from build123d import *

# Parameters (mm, degrees)
SKETCH1_W           = 155
SKETCH1_H           = 20
BOSS_EXTRUDE1_DEPTH = 40
CUT_EXTRUDE1_DEPTH  = 3
SKETCH4_W           = 78
SKETCH4_H           = 38
BOSS_EXTRUDE2_DEPTH = 20
FILLET1_R           = 5
SHELL2_START        = -10
SHELL2_DEPTH        = 18
SHELL2_START_2      = 2
SHELL2_2_DEPTH      = 3
CUT_EXTRUDE3_DEPTH  = 112.759787043
CUT_EXTRUDE4_REACH  = 110.311
SKETCH8_R           = 8
SKETCH9_R           = 2.05
CUT_EXTRUDE5_DEPTH  = 1.1


with BuildPart() as part:
    # Sketch1 → Boss-Extrude1 (new body)
    with BuildSketch(Plane(origin=(0, 0, 0), x_dir=(1, 0, 0), z_dir=(0, 1, 0))):
        Rectangle(SKETCH1_W, SKETCH1_H)
    extrude(amount=BOSS_EXTRUDE1_DEPTH)

    # Sketch2 → Cut-Extrude1 (cut)
    with BuildSketch(Plane.XZ):
        with BuildLine():
            Line((-71, -8), (71, -8))
            ThreePointArc((71, -8), (74.535533906, -6.535533906), (76, -3))
            Line((76, -3), (76, 3))
            ThreePointArc((76, 3), (74.535533906, 6.535533906), (71, 8))
            Line((71, 8), (-71, 8))
            ThreePointArc((-71, 8), (-74.535533906, 6.535533906), (-76, 3))
            Line((-76, 3), (-76, -3))
            ThreePointArc((-76, -3), (-74.535533906, -6.535533906), (-71, -8))
        make_face()
    extrude(amount=-CUT_EXTRUDE1_DEPTH, mode=Mode.SUBTRACT)

    # Sketch4 → Boss-Extrude2 (add)
    with BuildSketch(Plane.XY.offset(10)):
        with Locations((0, 59)):
            Rectangle(SKETCH4_W, SKETCH4_H)
    extrude(amount=-BOSS_EXTRUDE2_DEPTH)

    # Fillet1
    fillet1_edges = [part.edges().sort_by_distance(p)[0] for p in [
        (-77.5, 40, 0),
        (77.5, 40, 0),
        (-39, 78, 0),
        (39, 78, 0),
    ]]
    fillet(fillet1_edges, radius=FILLET1_R)

    # Shell2: read off the stored shape, not the designer's step
    # Shell2 outline → Shell2 (cut)
    with BuildSketch(Plane.XY.offset(SHELL2_START)):
        with BuildLine():
            Line((-75.5, 35), (-75.5, 5))
            Line((-75.5, 5), (75.5, 5))
            Line((75.5, 5), (75.5, 35))
            ThreePointArc((75.5, 35), (74.621320344, 37.121320344), (72.5, 38))
            Line((72.5, 38), (37, 38))
            Line((37, 38), (37, 73))
            ThreePointArc((37, 73), (36.121320344, 75.121320344), (34, 76))
            Line((34, 76), (-34, 76))
            ThreePointArc((-34, 76), (-36.121320344, 75.121320344), (-37, 73))
            Line((-37, 73), (-37, 38))
            Line((-37, 38), (-72.5, 38))
            ThreePointArc((-72.5, 38), (-74.621320344, 37.121320344), (-75.5, 35))
        make_face()
    extrude(amount=SHELL2_DEPTH, mode=Mode.SUBTRACT)

    # Shell2 2 outline → Shell2 2 (cut)
    with BuildSketch(Plane(origin=(0, 0, 0), x_dir=(1, 0, 0), z_dir=(0, 1, 0)).offset(SHELL2_START_2)):
        with BuildLine():
            Line((75.5, 10), (71, 10))
            ThreePointArc((71, 10), (73.394439545, 9.577739678), (75.5, 8.361902647))
            Line((75.5, 8.361902647), (75.5, 10))
        make_face()
        with BuildLine():
            ThreePointArc((-75.5, 8.361902647), (-73.394439545, 9.577739678), (-71, 10))
            Line((-71, 10), (-75.5, 10))
            Line((-75.5, 10), (-75.5, 8.361902647))
        make_face()
    extrude(amount=SHELL2_2_DEPTH, mode=Mode.SUBTRACT)

    # Sketch7 → Cut-Extrude3 (cut, through all)
    with BuildSketch(Plane.XY.offset(10)):
        with BuildLine():
            Line((-32.75, 18.5), (-32.75, 25.5))
            ThreePointArc((-32.75, 25.5), (-32.5, 25.75), (-32.25, 25.5))
            Line((-32.25, 25.5), (-32.25, 18.5))
            ThreePointArc((-32.25, 18.5), (-32.5, 18.25), (-32.75, 18.5))
        make_face()
        with BuildLine():
            Line((-31.75, 19.5), (-31.75, 24.5))
            ThreePointArc((-31.75, 24.5), (-31.5, 24.75), (-31.25, 24.5))
            Line((-31.25, 24.5), (-31.25, 19.5))
            ThreePointArc((-31.25, 19.5), (-31.5, 19.25), (-31.75, 19.5))
        make_face()
        with BuildLine():
            Line((-30.75, 20.5), (-30.75, 23.5))
            ThreePointArc((-30.75, 23.5), (-30.5, 23.75), (-30.25, 23.5))
            Line((-30.25, 23.5), (-30.25, 20.5))
            ThreePointArc((-30.25, 20.5), (-30.5, 20.25), (-30.75, 20.5))
        make_face()
        with BuildLine():
            Line((-33.25, 19.5), (-33.25, 24.5))
            ThreePointArc((-33.25, 24.5), (-33.5, 24.75), (-33.75, 24.5))
            Line((-33.75, 24.5), (-33.75, 19.5))
            ThreePointArc((-33.75, 19.5), (-33.5, 19.25), (-33.25, 19.5))
        make_face()
        with BuildLine():
            Line((-34.25, 20.5), (-34.25, 23.5))
            ThreePointArc((-34.25, 23.5), (-34.5, 23.75), (-34.75, 23.5))
            Line((-34.75, 23.5), (-34.75, 20.5))
            ThreePointArc((-34.75, 20.5), (-34.5, 20.25), (-34.25, 20.5))
        make_face()
    cut_extrude3 = extrude(amount=-CUT_EXTRUDE3_DEPTH, mode=Mode.SUBTRACT)

    # Mirror1: Cut-Extrude3 across plane
    add(cut_extrude3.mirror(Plane(origin=(0, 0, 0), x_dir=(0, 0, 1), z_dir=(1, 0, 0))), mode=Mode.SUBTRACT)

    # Sketch8 → Cut-Extrude4 (cut, up to next)
    with BuildSketch(Plane.XZ.offset(-3), mode=Mode.PRIVATE) as cut_extrude4_sk1:
        with Locations(Location((0, 0, 0), (0, 0, 90))):
            Circle(SKETCH8_R)
    cut_extrude4_tool1 = extrude(cut_extrude4_sk1.sketch, amount=-CUT_EXTRUDE4_REACH, mode=Mode.PRIVATE) & part.part
    add(cut_extrude4_tool1.solids().sort_by_distance((0, 3, 0))[0], mode=Mode.SUBTRACT)

    # Sketch9 → Cut-Extrude5 (cut)
    with BuildSketch(Plane.XZ.offset(-3)):
        with Locations(Location((70.75, 2.75, 0), (0, 0, 270))):
            Circle(SKETCH9_R)
        with Locations(Location((66.25, 2.75, 0), (0, 0, 270))):
            Circle(SKETCH9_R)
        with Locations(Location((66.25, -2.75, 0), (0, 0, 270))):
            Circle(SKETCH9_R)
        with Locations(Location((70.75, -2.75, 0), (0, 0, 270))):
            Circle(SKETCH9_R)
    cut_extrude5 = extrude(amount=-CUT_EXTRUDE5_DEPTH, mode=Mode.SUBTRACT)

    # Mirror2: Cut-Extrude5 across plane
    add(cut_extrude5.mirror(Plane(origin=(0, 0, 0), x_dir=(0, 0, 1), z_dir=(1, 0, 0))), mode=Mode.SUBTRACT)


solid = part.part
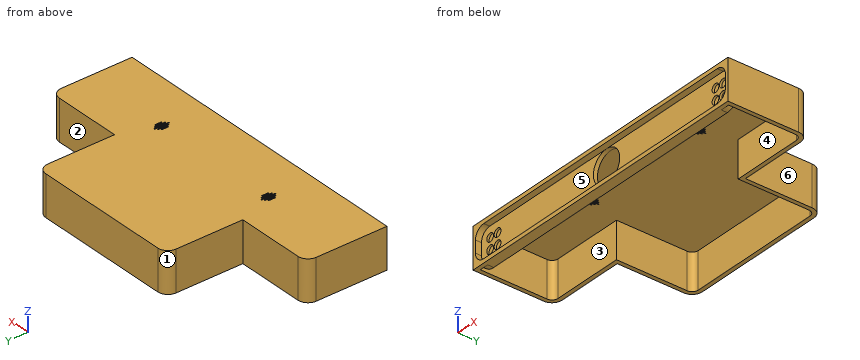
Geometry check sheet. Reference: the model listing, model coordinates, mm. Face numbers are marked on the shaded views. A direction names the side the tool comes from. Round coordinates to 2 decimals unless told otherwise and drop trailing zeros. Loops run counter-clockwise (first coordinate to the right, second up) from the corner with the lowest first, then second, coordinate; pieces in that order, holes last. Notation, with made-up numbers: (-24.5, 45.25) - (1.5, 45.25) arc R21 ccw to (1.5, 50.25) - close; hole circle Ø10 at (46, 10.25). An arc over 180 degrees is marked (long way). One line per question, with ' | ' between items. Start each with the question number.
1. Scan lines: line 1 (X direction, y = 18, z = -8); line 2 (Y direction, x = 52, z = -3.5); line 3 (X direction, y = 69, z = -6). Record each from-to range of solid material in increasing order. Write a range as [from, to].
2. Tool access check on the marked faces 4, 5 and 6. Record the directions out of +Z, -Z, +X, -X, +Y, -Y that give a thin tool (end or side, any length) a straight path to the whole face; none if there is none.
3. Draft check along X on the marked faces 1, 2 and 3. Enter one of: released by +X, released by -X, zero draft, split by the parting line, or undercut.
4. Cross-section at C-C on x = 61. Record the cut outline in (y, z).
5. Depth check by flat-ended pin: pin 1 (1.5 mm diameter, centred on x = -54, z = -2.5, fed in from -Y); pin 2 (4.5 mm diameter, centred on x = 70.75, z = 2.75, fed in from +Y); pin 3 (1.2 mm diameter, centred on x = -66, z = 3, fed in from -Y). Enter the tip coordinate at first touch or a pass-through.
6. Cross-section at A-A on x = -2. Record the cut outline in (y, z), then the cut area to 3 significant figures.
7. Cross-section at B-B on y = 55. Record the cut outline in (x, z), then the cut area to 3 significant figures.
Taken from the geometry:
1) line 1: [-77.5, -75.5], [75.5, 77.5] | line 2: [3, 5], [38, 40] | line 3: [-39, -37], [37, 39]
2) face 4: -Z | face 5: -Y | face 6: +Z, -Z, +X, +Y
3) face 1: released by -X | face 2: zero draft | face 3: undercut
4) outline: (0, -10) - (5, -10) - (5, 8) - (38, 8) - (38, -10) - (40, -10) - (40, 10) - (0, 10) - (0, 8) - (3, 8) - (3, -8) - (0, -8) - close
5) pin 1: y = 3 | pin 2: y = 40 | pin 3: y = 4.1
6) outline: (0, -10) - (5, -10) - (5, -7.75) - (3, -7.75) - (3, -8) - (0, -8) - close; (0, 8) - (3, 8) - (3, 7.75) - (5, 7.75) - (5, 8) - (76, 8) - (76, -10) - (78, -10) - (78, 10) - (0, 10) - close | area: 203 mm²
7) outline: (-39, -10) - (-37, -10) - (-37, 8) - (37, 8) - (37, -10) - (39, -10) - (39, 10) - (-39, 10) - close | area: 228 mm²
